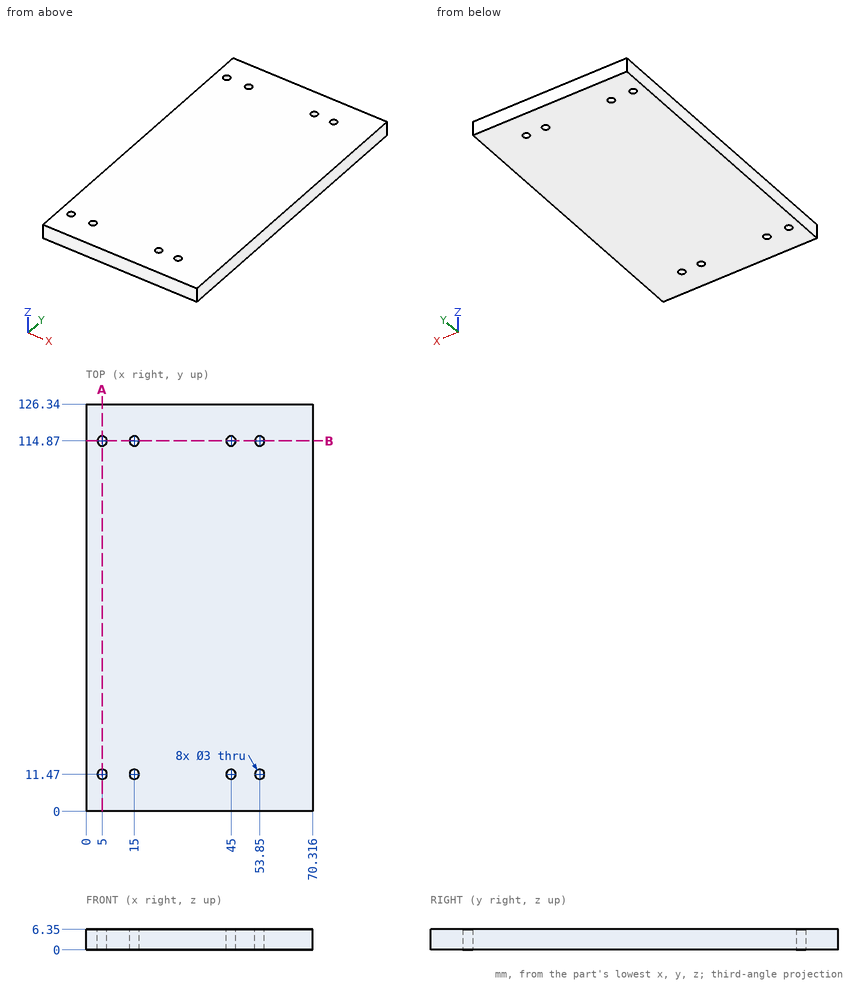
Source: three-view drawing plus pictorial views. Frame: mm from the lowest corner of the part. Coordinates: 2 decimals unless noted, no trailing zeros. Order: outer loops, then holes, each group sorted by start corner. A loop starts at its lowest first (then second) coordinate and runs counter-clockwise, first axis right, second up. Notation, with made-up numbers: M 47.5,-16 L 66.5,-16 A15 ccw 66.5,-8 Z; hole C 17,-8.75 d7. An arc over 180 degrees is marked long. Write each question's results on one line, items separated by ' | '. Start each with the question number.
1. Material intervals for L1, parallel to Y at x = 5, z = 4.5; L2, parallel to X at y = 12.5, z = 4.5 (1 decimal); L3, parallel to Y at x = 5.5, z = 5.75 (1 decimal), sorted ascending.
2. Section A-A, the plane x = 5. Return the cut outline in (y, z), then the cut area to 3 significant figures.
3. Section B-B, the plane y = 114.87. State how many separate pieces and enclosed holes the cut face has, then the cut area to 3 significant figures.
Solution:
1) L1: 0 to 9.97, 12.97 to 113.37, 116.37 to 126.34 | L2: 0 to 3.9, 6.1 to 13.9, 16.1 to 43.9, 46.1 to 52.8, 54.9 to 70.3 | L3: 0 to 10.1, 12.9 to 113.5, 116.3 to 126.3
2) outline: M 0,0 L 9.97,0 L 9.97,6.35 L 0,6.35 Z; M 12.97,0 L 113.37,0 L 113.37,6.35 L 12.97,6.35 Z; M 116.37,0 L 126.34,0 L 126.34,6.35 L 116.37,6.35 Z | area: 764 mm²
3) separate pieces: 5 | enclosed holes: 0 | area: 370 mm²
